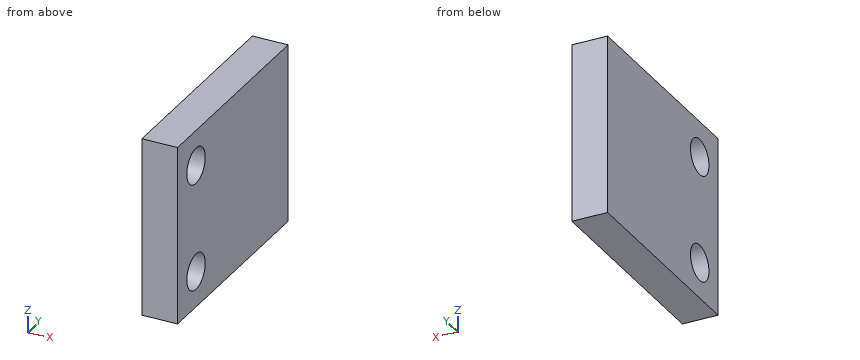
Autodesk Inventor part; units mm, degrees
ref_plane "YZ Plane" through (0, 0, 0) normal (1, 0, 0) x (0, 1, 0)
ref_plane "XZ Plane" through (0, 0, 0) normal (0, 1, 0) x (-1, 0, 0)
ref_plane "XY Plane" through (0, 0, 0) normal (0, 0, 1) x (1, 0, 0)
sketch "スケッチ1" plane through (0, 0, 0) normal (0, 0, 1) x (1, 0, 0)
  line L0 (0, 0) -> (5, 0)
  line L1 (5, 0) -> (5, 30)
  line L2 (5, 30) -> (0, 30)
  line L3 (0, 30) -> (0, 0)
  line L4 (5, 30) -> (15, 30)
  line L5 (15, 30) -> (15, 0)
  line L6 (15, 0) -> (5, 0)
  line L7 (5, 0) -> (5, 30)
  dimension "d0" = 30
  dimension "d1" = 5
  dimension "d2" = 30
  dimension "d3" = 10
extrude "押し出し1" add sketch "スケッチ1" along normal blind 5
sketch "スケッチ2" plane through (0, 0, 5) normal (0, 0, 1) x (1, 0, 0)
  line L0 (15, 0) -> (15, 30)
  line L1 (0, 0) -> (15, 0)
  line L2 (15, 30) -> (5, 30)
  line L3 (5, 30) -> (5, 0)
  line L4 (5, 0) -> (15, 0)
  line L5 (15, 0) -> (15, 30)
  point P0 (10, 21)
  point P1 (10, 9)
  dimension "d6" = 10
  dimension "d7" = 5
  dimension "d8" = 9
  dimension "d9" = 9
  dimension "d10" = 5
hole "穴1" at (10, 21, 5) at (10, 9, 5) direction (0, 0, -1) diameter 5 depth 8
sketch "スケッチ3" plane through (0, 0, 5) normal (0, 0, 1) x (1, 0, 0)
  line L0 (15, 30) -> (0, 30)
  line L1 (0, 0) -> (15, 0)
  line L2 (0, 30) -> (5, 30)
  line L3 (5, 30) -> (5, 0)
  line L4 (5, 0) -> (0, 0)
  line L5 (0, 0) -> (0, 30)
  dimension "d18" = 5
extrude "押し出し2" add sketch "スケッチ3" along normal blind 30
sketch "スケッチ4" plane through (5, 0, 5) normal (1, 0, 0) x (0, 0, -1)
  line L0 (-30, 0) -> (-30, 30)
  line L1 (0, 0) -> (-30, 0)
  line L2 (5, 0) -> (5, 30)
  point P0 (-20, 5)
  point P1 (-5, 5)
  dimension "d21" = 15
  dimension "d22" = 10
  dimension "d23" = 5
  dimension "d24" = 5
  dimension "d25" = 10
hole "穴2" at (5, 5, 25) at (5, 5, 10) direction (-1, 0, 0) diameter 5 depth 8
sketch "スケッチ5" plane through (5, 0, 5) normal (1, 0, 0) x (0, 0, -1)
  line L0 (5, 30) -> (-30, 30)
  line L1 (-30, 30) -> (-25, 30)
  line L2 (-25, 30) -> (-25, 0)
  line L3 (-25, 0) -> (-30, 0)
  line L4 (-30, 0) -> (-30, 30)
  line L5 (0, 0) -> (0, 30)
  circle A0 centre (-5, 5) radius 2.5
  circle A1 centre (-20, 5) radius 2.5
  point P0 (5, 0)
  dimension "d33" = 5
  dimension "d34" = 5
extrude "押し出し3" cut sketch "スケッチ5" against normal through all contours L2 L3 L4 L0
sketch "スケッチ6" plane through (0, 0, 0) normal (0, 0, -1) x (-1, 0, 0)
  line L0 (-35.4456, 44.1041) -> (17.4783, 44.1041)
  line L1 (17.4783, 44.1041) -> (17.4783, -11.5216)
  line L2 (17.4783, -11.5216) -> (-35.4456, -11.5216)
  line L3 (-35.4456, -11.5216) -> (-35.4456, 44.1041)
  point P0 (0, 0)
extrude "押し出し4" cut sketch "スケッチ6" against normal blind 5
equation "\"d34\" = d33"
properties part number "BP_BOX-Support-Bar-Connect2"
Read the model definition and answer for the solid it produces. Units are mm, in the model's axes. Round coordinates to 2 decimals unless told otherwise and drop trailing zeros. Order: outer loops, then holes, each group sorted by start corner. A loop starts at its lowest first (then second) coordinate and runs counter-clockwise, first axis right, second up.
1) Straight lines are drawn through the part: L1, parallel to Z at x = 2.35, y = 5; L2, parallel to Y at x = 3.25, z = 25; L3, parallel to Z at x = 4.45, y = 7. For each, find the intervals that lie inside material, in ascending order.
2) The part is cut by section A-A on y = 5. Write down the section's boundary in (x, z).
3) The part is cut by section B-B on z = 10. Write down the section's boundary in (x, y), plus the area to 3 significant figures.
4) The part is cut by section C-C on x = 3.25. Write down the section's boundary in (y, z), plus the area to 3 significant figures.
5) The part is cut by section D-D on z = 24. Write down the section's boundary in (x, y), plus the area to 3 significant figures.
Resolved:
1. L1: z = 5 to 7.5, 12.5 to 22.5, 27.5 to 30
1. L2: y = 0 to 2.5, 7.5 to 30
1. L3: z = 5 to 8.5, 11.5 to 23.5, 26.5 to 30
2. outline: (0, 5) - (5, 5) - (5, 7.5) - (0, 7.5) - close; (0, 12.5) - (5, 12.5) - (5, 22.5) - (0, 22.5) - close; (0, 27.5) - (5, 27.5) - (5, 30) - (0, 30) - close
3. outline: (0, 0) - (5, 0) - (5, 2.5) - (0, 2.5) - close; (0, 7.5) - (5, 7.5) - (5, 30) - (0, 30) - close
3. area: 125 mm2
4. outline: (0, 5) - (30, 5) - (30, 30) - (0, 30) - close; hole circle Ø5 at (5, 10); hole circle Ø5 at (5, 25)
4. area: 711 mm2
5. outline: (0, 0) - (5, 0) - (5, 2.71) - (0, 2.71) - close; (0, 7.29) - (5, 7.29) - (5, 30) - (0, 30) - close
5. area: 127 mm2
